The listing builds one solid part. Answer for the finished solid, in the listing's coordinates (mm). Round coordinates to 2 decimals unless told otherwise and drop trailing zeros. Write each loop counter-clockwise with the first axis right and the second up, starting at its lowest first coordinate (ties: lowest second). Pieces come first, ordered by that corner, then holes. Notation, with made-up numbers: M 10.25,31 L 68.25,31 A29 cw 68.25,57 Z; hole C -18,36 d8. An arc over 180 degrees is marked long. One line per item, written item: value. Start each with the question number.
(1) Section A-A (x = 0) is taken. Determine the outline of the cut face in (y, z).
(2) Section D-D (x = 22) is taken. Determine the outline of the cut face in (y, z), plus the area to 3 significant figures.
(3) Given P1, Ø3.5, axis at x = -17, z = 29.44, coming from the +Y side; P2, Ø2, axis at x = -35, z = 1, coming from the +Y side, each flat-ended and moving along its own axis, determine where each tip first touches the part or whether it passes through.
(4) Section B-B (z = 12) is taken. Determine the outline of the cut face in (x, y).
(5) Section C-C (y = 3.2) is taken. State how many separate pieces and enclosed holes the cut face has, plus the area to 3 significant figures.
(6) Consider probe 1 along X at (y, z) = (4.85, 17); probe 2 along X at (y, z) = (0.35, -16); probe 3 along Z at (x, y) = (-18.5, 4.8). Determine where each line is inside the solid, lowest interval first.
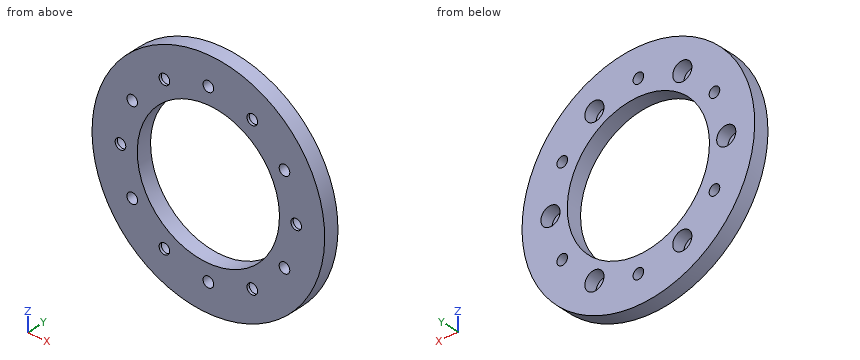
```python
from build123d import *

# Parameters (mm, degrees)
SKETCH_1_R          = 45
SKETCH_1_R_2        = 2.05
SKETCH_1_R_3        = 27.5
EXTRUDE_1_DEPTH     = 6
SKETCH_2_R          = 3.7
CUT_EXTRUDE_1_DEPTH = 5


with BuildPart() as part:
    # 草图1 → 凸台-拉伸1 (new body)
    with BuildSketch(Plane(origin=(0, 0, 0), x_dir=(1, 0, 0), z_dir=(0, 1, 0))):
        with Locations(Location((0, 0, 0), (0, 0, 270))):
            Circle(SKETCH_1_R)
        with Locations(Location((34, 0, 0), (0, 0, 270))):
            Circle(SKETCH_1_R_2, mode=Mode.SUBTRACT)
        with Locations(Location((29.444863729, -17, 0), (0, 0, 270))):
            Circle(SKETCH_1_R_2, mode=Mode.SUBTRACT)
        with Locations(Location((17, -29.444863729, 0), (0, 0, 270))):
            Circle(SKETCH_1_R_2, mode=Mode.SUBTRACT)
        with Locations(Location((0, -34, 0), (0, 0, 270))):
            Circle(SKETCH_1_R_2, mode=Mode.SUBTRACT)
        with Locations(Location((-17, -29.444863729, 0), (0, 0, 270))):
            Circle(SKETCH_1_R_2, mode=Mode.SUBTRACT)
        with Locations(Location((-29.444863729, -17, 0), (0, 0, 270))):
            Circle(SKETCH_1_R_2, mode=Mode.SUBTRACT)
        with Locations(Location((-34, 0, 0), (0, 0, 270))):
            Circle(SKETCH_1_R_2, mode=Mode.SUBTRACT)
        with Locations(Location((-29.444863729, 17, 0), (0, 0, 270))):
            Circle(SKETCH_1_R_2, mode=Mode.SUBTRACT)
        with Locations(Location((-17, 29.444863729, 0), (0, 0, 270))):
            Circle(SKETCH_1_R_2, mode=Mode.SUBTRACT)
        with Locations(Location((0, 34, 0), (0, 0, 270))):
            Circle(SKETCH_1_R_2, mode=Mode.SUBTRACT)
        with Locations(Location((17, 29.444863729, 0), (0, 0, 270))):
            Circle(SKETCH_1_R_2, mode=Mode.SUBTRACT)
        with Locations(Location((29.444863729, 17, 0), (0, 0, 270))):
            Circle(SKETCH_1_R_2, mode=Mode.SUBTRACT)
        with Locations(Location((0, 0, 0), (0, 0, 270))):
            Circle(SKETCH_1_R_3, mode=Mode.SUBTRACT)
    extrude(amount=EXTRUDE_1_DEPTH)

    # 草图2 → 切除-拉伸1 (cut)
    with BuildSketch(Plane(origin=(0, 6, 0), x_dir=(1, 0, 0), z_dir=(0, 1, 0))):
        with Locations(Location((34, 0, 0), (0, 0, 270))):
            Circle(SKETCH_2_R)
        with Locations(Location((17, -29.444863729, 0), (0, 0, 270))):
            Circle(SKETCH_2_R)
        with Locations(Location((-17, -29.444863729, 0), (0, 0, 270))):
            Circle(SKETCH_2_R)
        with Locations(Location((-34, 0, 0), (0, 0, 270))):
            Circle(SKETCH_2_R)
        with Locations(Location((-17, 29.444863729, 0), (0, 0, 270))):
            Circle(SKETCH_2_R)
        with Locations(Location((17, 29.444863729, 0), (0, 0, 270))):
            Circle(SKETCH_2_R)
    extrude(amount=-CUT_EXTRUDE_1_DEPTH, mode=Mode.SUBTRACT)


solid = part.part
```
Recorded:
1. outline: M 0,-45 L 6,-45 L 6,-36.05 L 0,-36.05 Z; M 0,-31.95 L 6,-31.95 L 6,-27.5 L 0,-27.5 Z; M 0,27.5 L 6,27.5 L 6,31.95 L 0,31.95 Z; M 0,36.05 L 6,36.05 L 6,45 L 0,45 Z
2. outline: M 0,-39.26 L 6,-39.26 L 6,-16.5 L 0,-16.5 Z; M 0,16.5 L 6,16.5 L 6,39.26 L 0,39.26 Z
2. area: 273 mm2
3. P1: passes through
3. P2: stops at y = 1
4. outline: M -43.37,0 L -24.74,0 L -24.74,6 L -43.37,6 Z; M 24.74,0 L 43.37,0 L 43.37,6 L 24.74,6 Z
5. separate pieces: 1
5. enclosed holes: 13
5. area: 3,650 mm2
6. probe 1: x = -41.67 to -31.49, -27.39 to -21.62, 21.62 to 27.39, 31.49 to 41.67
6. probe 2: x = -42.06 to -31.23, -27.66 to -22.37, 22.37 to 27.66, 31.23 to 42.06
6. probe 3: z = -41.02 to -32.83, -26.06 to -20.35, 20.35 to 26.06, 32.83 to 41.02
